Input: part model. Units: mm. Frame: model coordinates. Coordinates: 2 decimals unless noted, no trailing zeros. Loops run counter-clockwise (first coordinate to the right, second up) from the corner with the lowest first, then second, coordinate; pieces in that order, holes last.
(1) Section D-D, the plane x = -1685.3. Return loops of the section in (y, z).
(2) Contact query for flat-ended pins moving along their axis: P1, Ø5, axis at x = -1663.3, z = 135.22, coming from the +Y side; P2, Ø6, axis at x = -1672.5, z = 112, coming from the -Y side; P3, Ø1, axis at x = -1664.5, y = 2.5, coming from the +Z side. Output: stop coordinate, or through.
(3) Section B-B, the plane x = -1661. Return loops of the section in (y, z).
(4) Section A-A, the plane z = 134.5. Return loops of the section in (x, y).
(5) Mould query, pull axis X, two halves, no side actions, for faces 1 (the face through (-1675.651, 1.479, 125.846)), 2 (the face through (-1671, 0, 129)), 3 (the face through (-1665.418, 1.479, 120.068)). Classes: released by +X, released by -X, zero draft, split by the parting line, or undercut.
(6) Line query: L1, parallel to Z at x = -1663.3, y = 2.05; L2, parallel to Z at x = -1664, y = 1.7; L3, parallel to X at y = 0.2, z = 108.5. Output: solid intervals per line, ascending.
```python
from build123d import *

# Parameters (mm, degrees)
SZKIC1_R                    = 4
DODANIE_WYCI_GNI_CIE1_DEPTH = 3


with BuildPart() as part:
    # Szkic1 → Dodanie-wyciągnięcie1 (new body)
    with BuildSketch(Plane(origin=(0, 0, 0), x_dir=(1, 0, 0), z_dir=(0, 1, 0))):
        with BuildLine():
            Line((-1665.878196442, -141.728418885), (-1690.824706662, -131.845523163))
            ThreePointArc((-1690.824706662, -131.845523163), (-1692.780138286, -130.901827995), (-1694.578843612, -129.685714286))
            Line((-1694.578843612, -129.685714286), (-1693.032369677, -127.721428571))
            ThreePointArc((-1693.032369677, -127.721428571), (-1675.478571429, -125.632369677), (-1677.567630323, -108.078571429))
            Line((-1677.567630323, -108.078571429), (-1676.021156388, -106.114285714))
            ThreePointArc((-1676.021156388, -106.114285714), (-1674.416864421, -107.577337555), (-1673.04059946, -109.256673186))
            Line((-1673.04059946, -109.256673186), (-1657.578946415, -131.186955563))
            ThreePointArc((-1657.578946415, -131.186955563), (-1657.8, -139.550635095), (-1665.878196442, -141.728418885))
        make_face()
        with Locations((-1663.3, -135.220508076)):
            Circle(SZKIC1_R, mode=Mode.SUBTRACT)
    extrude(amount=DODANIE_WYCI_GNI_CIE1_DEPTH)


solid = part.part
```
Report:
1. outline: (0, 130.4) - (3, 130.4) - (3, 134.03) - (0, 134.03) - close
2. P1: passes through
2. P2: stops at y = 0
2. P3: stops at z = 142.19
3. outline: (0, 126.33) - (3, 126.33) - (3, 131.95) - (0, 131.95) - close; (0, 138.49) - (3, 138.49) - (3, 141.83) - (0, 141.83) - close
4. outline: (-1684.12, 0) - (-1667.23, 0) - (-1667.23, 3) - (-1684.12, 3) - close; (-1659.37, 0) - (-1656.34, 0) - (-1656.34, 3) - (-1659.37, 3) - close
5. face 1: undercut
5. face 2: zero draft
5. face 3: released by +X
6. L1: z = 123.07 to 131.22, 139.22 to 142.22
6. L2: z = 122.08 to 131.28, 139.16 to 142.19
6. L3: x = -1677.06 to -1673.61
